Autodesk Inventor part; units mm, degrees
ref_plane "YZ Plane" through (0, 0, 0) normal (1, 0, 0) x (0, 1, 0)
ref_plane "XZ Plane" through (0, 0, 0) normal (0, 1, 0) x (-1, 0, 0)
ref_plane "XY Plane" through (0, 0, 0) normal (0, 0, 1) x (1, 0, 0)
sketch "Sketch1" plane through (0, 0, 0) normal (0, 0, 1) x (1, 0, 0)
  line L0 (0, 0) -> (25.4, 0)
  line L1 (25.4, 0) -> (25.4, 25.4)
  line L2 (25.4, 25.4) -> (0, 25.4)
  line L3 (0, 25.4) -> (0, 0)
  line L4 (3.175, 3.175) -> (22.225, 3.175)
  line L5 (22.225, 3.175) -> (22.225, 22.225)
  line L6 (22.225, 22.225) -> (3.175, 22.225)
  line L7 (3.175, 22.225) -> (3.175, 3.175)
  dimension "d0" = 25.4
  dimension "d1" = 25.4
  dimension "d2" = 3.175
extrude "Extrusion1" add sketch "Sketch1" against normal blind 990.6
sketch "Sketch3" plane through (0, 25.4, 0) normal (0, 1, 0) x (1, 0, 0)
  line L0 (25.4, 0) -> (0, 0)
  point P0 (12.7, 12.7)
  point P1 (12.7, 38.1)
  dimension "d24" = 12.7
  dimension "d25" = 25.4
hole "Hole3" at (12.7, 25.4, -12.7) at (12.7, 25.4, -38.1) direction (0, -1, 0) diameter 6.35 depth 25.4 tip angle 118
sketch "Sketch4" plane through (0, 0, 0) normal (-1, 0, 0) x (0, 0, 1)
  line L0 (0, 25.4) -> (0, 0)
  point P0 (-12.7, 12.7)
  point P1 (-38.1, 12.7)
  dimension "d33" = 12.7
  dimension "d34" = 25.4
hole "Hole4" at (0, 12.7, -12.7) at (0, 12.7, -38.1) direction (1, 0, 0) diameter 6.35 depth 25.4 tip angle 118
sketch "Sketch5" plane through (25.4, 0, 0) normal (1, 0, 0) x (0, 0, -1)
  line L0 (0, 0) -> (0, 25.4)
  point P0 (317.5, 12.7)
  point P1 (342.9, 12.7)
  point P2 (368.3, 12.7)
  point P3 (647.7, 12.7)
  point P4 (673.1, 12.7)
  point P5 (698.5, 12.7)
  point P6 (812.8, 12.7)
  point P7 (508, 12.7)
  point P8 (203.2, 12.7)
  point P9 (977.9, 12.7)
  point P10 (952.5, 12.7)
  dimension "d42" = 317.5
  dimension "d43" = 25.4
  dimension "d44" = 25.4
  dimension "d45" = 25.4
  dimension "d46" = 25.4
  dimension "d47" = 279.4
  dimension "d55" = 114.3
  dimension "d56" = 139.7
  dimension "d57" = 114.3
  dimension "d58" = 25.4
  dimension "d59" = 139.7
hole "Hole5" at (25.4, 12.7, -317.5) at (25.4, 12.7, -342.9) at (25.4, 12.7, -368.3) at (25.4, 12.7, -647.7) at (25.4, 12.7, -673.1) at (25.4, 12.7, -698.5) at (25.4, 12.7, -203.2) at (25.4, 12.7, -508) at (25.4, 12.7, -812.8) at (25.4, 12.7, -952.5) at (25.4, 12.7, -977.9) direction (-1, 0, 0) diameter 6.35 depth 25.4 tip angle 118
properties part number "towertallfrontthing"
Read the model definition and answer for the solid it produces. Units are mm, in the model's axes. A direction names the side the tool comes from. Give positions to 0.01 mm unless a question says otherwise; leave off trailing zeros. Write each loop counter-clockwise with the first axis right and the second up, starting at its lowest first coordinate (ties: lowest second). Pieces come first, ordered by that corner, then holes. Notation, with made-up numbers: (12.25, 87.25) -> (22.25, 87.25) arc R21 cw to (22.25, 110.25) -> close; hole circle Ø5 at (53.25, 79). An arc over 180 degrees is marked (long way). Answer in a Markdown table with one row per item.
1) Section A-A on z = -302 is taken. Give the vertices of the cut face in (x, y) (3 decimals).
Results list:
| item | result |
|---|---|
| outline | (0, 0) -> (25.4, 0) -> (25.4, 25.4) -> (0, 25.4) -> close; hole (3.175, 3.175) -> (22.225, 3.175) -> (22.225, 22.225) -> (3.175, 22.225) -> close |
2) A tool of negligible diameter and unlimited length cuts with its end or side. For faces 1 (the flat face through (25.4, 13, -488)), 2 (the flat face through (13, 22.225, -488)), from which of +Z, -Z, +X, -X, +Y, -Y can it reach the whole face along a straight path? Write none if from no direction.
Results list:
| item | result |
|---|---|
| face 1 | +Z, -Z, +X, +Y, -Y |
| face 2 | +Z, -Z |
3) This flat-tipped pin is pushed along its axis until it touches: pin 1 Ø5 at (y, z) = (12.7, -342.9) entering from -X. Where does it stop, or does it pass through?
Results list:
| item | result |
|---|---|
| pin 1 | through |
4) Straight lines are drawn through the part: line 1 (Y direction, x = 19.25, z = -774.5) (3 decimals); line 2 (Y direction, x = 1.4, z = -812.8) (3 decimals). For each, find the intervals that lie inside material, in ascending order. Write a range as [from, to].
Results list:
| item | result |
|---|---|
| line 1 | [0, 3.175], [22.225, 25.4] |
| line 2 | [0, 9.525], [15.875, 25.4] |
5) Determine the mould class of faces 3 (the flat face through (3.175, 13, -488)), 4 (the flat face through (0, 13, -488)), 5 (the flat face through (13, 0, -488)) for opening direction X: released by +X, released by -X, zero draft, split by the parting line, or undercut.
Results list:
| item | result |
|---|---|
| face 3 | undercut |
| face 4 | released by -X |
| face 5 | zero draft |
